from build123d import *

# Parameters (mm, degrees)
DODANIE_WYCI_GNI_CIE1_DEPTH = 15


with BuildPart() as part:
    # Szkic1 → Dodanie-wyciągnięcie1 (new body)
    with BuildSketch(Plane.XY):
        Polygon((20.5, 0), (-20.5, 0), (-23.5, 0), (-23.5, 10), (-20.5, 10), (-20.5, 3), (-17.35, 3), (-17.35, 10), (-14.351157044, 10), (-14.351157044, 3), (14.351157044, 3), (14.351157044, 10), (17.35, 10), (17.35, 3), (20.5, 3), (20.5, 10), (23.5, 10), (23.5, 0), align=None)
    extrude(amount=DODANIE_WYCI_GNI_CIE1_DEPTH)


solid = part.part
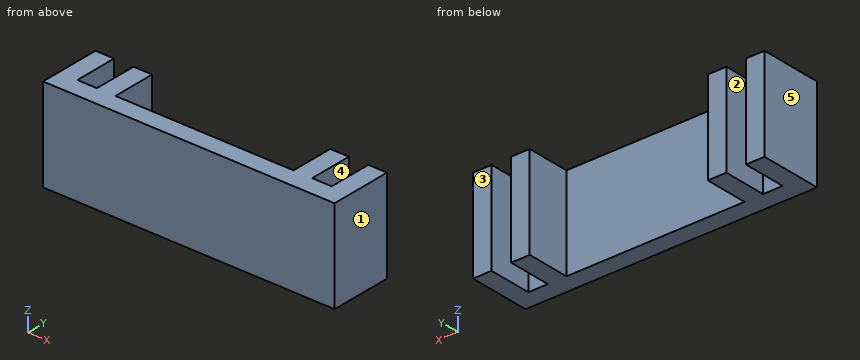
Input: part model. Units: mm. Frame: model coordinates. Face numbers are marked on the shaded views. A direction names the side the tool comes from. Coordinates: 2 decimals unless noted, no trailing zeros. Loops run counter-clockwise (first coordinate to the right, second up) from the corner with the lowest first, then second, coordinate; pieces in that order, holes last. Notation, with made-up numbers: (-17, -2) -> (15, -2) arc R19 cw to (15, 32) -> close; hole circle Ø4 at (53, -9). An arc over 180 degrees is marked (long way). Write item = value, one per line. Start each with the question number.
Item 1: Material intervals for line 1 (X direction, y = 6.5, z = 10); line 2 (Y direction, x = -18, z = 3.75), sorted ascending.
Item 2: Cut plane B-B, the plane z = 6.5. Return loops of the section in (x, y).
Item 3: Reachability of the marked faces 1 and 2 from +Z, -Z, +X, -X, +Y, -Y: full face, straight path, thin tool, end or side. Return the list, or none.
Item 4: Cut plane A-A, the plane y = 4.5. Return loops of the section in (x, z), plus the area to 3 significant figures.
Item 5: Cut plane C-C, the plane x = -18. Return loops of the section in (y, z).
Item 6: Mould query, pull axis X, two halves, no side actions, for the marked faces 3, 4 and 5. Classes: pulls with the +X half, pulls with the -X half, needs draft (parallel to the pull), parting line crosses it, or undercut.
Item 7: First-contact query: P1, Ø7.5, axis at x = -5.5, z = 10.5, coming from the +Y side. Flat tip, straight axial feed; report the tip coordinate or a pass-through.
Ans:
q1.line_1 = -23.5 to -20.5, -17.35 to -14.35, 14.35 to 17.35, 20.5 to 23.5
q1.line_2 = 0 to 3
q2.outline = (-23.5, 0) -> (23.5, 0) -> (23.5, 10) -> (20.5, 10) -> (20.5, 3) -> (17.35, 3) -> (17.35, 10) -> (14.35, 10) -> (14.35, 3) -> (-14.35, 3) -> (-14.35, 10) -> (-17.35, 10) -> (-17.35, 3) -> (-20.5, 3) -> (-20.5, 10) -> (-23.5, 10) -> close
q3.face_1 = +Z, -Z, +X, +Y, -Y
q3.face_2 = +Z, -Z, +Y
q4.outline = (-23.5, 0) -> (-20.5, 0) -> (-20.5, 15) -> (-23.5, 15) -> close; (-17.35, 0) -> (-14.35, 0) -> (-14.35, 15) -> (-17.35, 15) -> close; (14.35, 0) -> (17.35, 0) -> (17.35, 15) -> (14.35, 15) -> close; (20.5, 0) -> (23.5, 0) -> (23.5, 15) -> (20.5, 15) -> close
q4.area = 180 mm²
q5.outline = (0, 0) -> (3, 0) -> (3, 15) -> (0, 15) -> close
q6.face_3 = needs draft
q6.face_4 = undercut
q6.face_5 = pulls with the -X half
q7.P1 = 3
